The listing builds one solid part. Answer for the finished solid, in the listing's coordinates (mm). A direction names the side the tool comes from. Round coordinates to 2 decimals unless told otherwise and drop trailing zeros. Write each loop counter-clockwise with the first axis right and the second up, starting at its lowest first coordinate (ties: lowest second). Pieces come first, ordered by that corner, then holes.
Item 1: Find section A-A on x = 6. Give the vertices of the cut face in (y, z), then the cut area to 3 significant figures.
Item 2: Find section D-D on y = 25. Give the vertices of the cut face in (x, z), then the cut area to 3 significant figures.
Item 3: Find section C-C on z = 12.5. Give the vertices of the cut face in (x, y).
Item 4: For a pull along X with two mould halves and no side action, classify faces 6 (the face through (0, -1, 83)), 7 (the face through (44.615, 22.504, -0.986)), 8 (the face through (44, -4, 62)) as +X half, -X half, draft (parallel to the pull), parting line (faces both ways), or undercut.
Item 5: A tool of negligible diameter and unlimited length cuts with its end or side. For faces 1 (the face through (34, 13, 128)), 2 (the face through (82.125, 24.119, -0.986)), 3 (the face through (44, 60, 126)), 4 (the face through (62.169, 35.407, 126.028)), 5 (the face through (24, 30, 124)), from which of +Z, -Z, +X, -X, +Y, -Y can it reach the whole face along a straight path? Write none if from no direction.
Item 6: Each of these flat-tipped pins is pushed along its axis until it touches: pin 1 (5.5 mm diameter, centred on x = 6, z = 12.5, fed in from +Y); pin 2 (1.6 mm diameter, centred on x = 13, z = -1, fed in from +Y). Where does it stop, or does it pass through?
Item 7: Find the intervals of material crossed by probe 1 along X at (y, z) = (-3.15, 12.5); probe 2 along Z at (x, y) = (15, 33.5); probe 3 along X at (y, z) = (-2, 12) (3 decimals), in increasing order.
Item 8: Find section B-B on y = 6. Give the vertices of the cut face in (x, z).
```python
from build123d import *

# Parameters (mm, degrees)
SKETCH1_R           = 2.3
BOSS_EXTRUDE1_DEPTH = 2
SKETCH2_W           = 90
SKETCH2_H           = 4
BOSS_EXTRUDE2_DEPTH = 128
SKETCH3_W           = 90
SKETCH3_H           = 4
BOSS_EXTRUDE3_DEPTH = 60
SKETCH4_R           = 18
CUT_EXTRUDE1_DEPTH  = 60
SKETCH5_R           = 2.3
CUT_EXTRUDE2_DEPTH  = 60


with BuildPart() as part:
    # Sketch1 → Boss-Extrude1 (new body)
    with BuildSketch(Plane.XY):
        with BuildLine():
            Line((0, 0), (0, 40))
            Line((0, 40), (27.5, 40))
            ThreePointArc((27.5, 40), (45, 22.5), (62.5, 40))
            Line((62.5, 40), (90, 40))
            Line((90, 40), (90, 0))
            Line((90, 0), (90, -4))
            Line((90, -4), (0, -4))
            Line((0, -4), (0, 0))
        make_face()
        with Locations((10, 25)):
            Circle(SKETCH1_R, mode=Mode.SUBTRACT)
        with Locations((80, 25)):
            Circle(SKETCH1_R, mode=Mode.SUBTRACT)
    extrude(amount=-BOSS_EXTRUDE1_DEPTH)

    # Sketch2 → Boss-Extrude2 (add)
    with BuildSketch(Plane.XY):
        with Locations((45, -2)):
            Rectangle(SKETCH2_W, SKETCH2_H)
    extrude(amount=BOSS_EXTRUDE2_DEPTH)

    # Sketch3 → Boss-Extrude3 (add)
    with BuildSketch(Plane(origin=(0, 0, 0), x_dir=(1, 0, 0), z_dir=(0, 1, 0))):
        with Locations((45, -126)):
            Rectangle(SKETCH3_W, SKETCH3_H)
    extrude(amount=BOSS_EXTRUDE3_DEPTH)

    # Sketch4 → Cut-Extrude1 (cut)
    with BuildSketch(Plane.XY.offset(128)):
        with Locations((45, 30)):
            Circle(SKETCH4_R)
    extrude(amount=-CUT_EXTRUDE1_DEPTH, mode=Mode.SUBTRACT)

    # Sketch5 → Cut-Extrude2 (cut)
    with BuildSketch(Plane(origin=(0, 0, 0), x_dir=(1, 0, 0), z_dir=(0, 1, 0))):
        with Locations(Location((6, -12.5, 0), (0, 0, 270))):
            Circle(SKETCH5_R)
        with Locations(Location((84, -12.5, 0), (0, 0, 270))):
            Circle(SKETCH5_R)
    extrude(amount=-CUT_EXTRUDE2_DEPTH, mode=Mode.SUBTRACT)


solid = part.part
```
Check values:
1. outline: (-4, -2) - (40, -2) - (40, 0) - (0, 0) - (0, 10.2) - (-4, 10.2) - close; (-4, 14.8) - (0, 14.8) - (0, 124) - (60, 124) - (60, 128) - (-4, 128) - close
1. area: 822 mm2
2. outline: (0, -2) - (7.7, -2) - (7.7, 0) - (0, 0) - close; (0, 124) - (27.71, 124) - (27.71, 128) - (0, 128) - close; (12.3, -2) - (35.99, -2) - (35.99, 0) - (12.3, 0) - close; (54.01, -2) - (77.7, -2) - (77.7, 0) - (54.01, 0) - close; (62.29, 124) - (90, 124) - (90, 128) - (62.29, 128) - close; (82.3, -2) - (90, -2) - (90, 0) - (82.3, 0) - close
2. area: 347 mm2
3. outline: (0, -4) - (3.7, -4) - (3.7, 0) - (0, 0) - close; (8.3, -4) - (81.7, -4) - (81.7, 0) - (8.3, 0) - close; (86.3, -4) - (90, -4) - (90, 0) - (86.3, 0) - close
4. face 6: -X half
4. face 7: undercut
4. face 8: draft
5. face 1: +Z, +X, -X, +Y, -Y
5. face 2: -Z
5. face 3: +Z, -Z, +X, -X, +Y
5. face 4: +Z
5. face 5: +X, -X, +Y
6. pin 1: stops at y = 0
6. pin 2: stops at y = 40
7. probe 1: x = 0 to 3.7, 8.3 to 81.7, 86.3 to 90
7. probe 2: z = -2 to 0, 124 to 128
7. probe 3: x = 0 to 3.755, 8.245 to 81.755, 86.245 to 90
8. outline: (0, -2) - (90, -2) - (90, 0) - (0, 0) - close; (0, 124) - (90, 124) - (90, 128) - (0, 128) - close
